Check sheet for the modelled part. Datum: model origin and axes. Units: mm. A direction names the side the tool comes from. Round coordinates to 2 decimals unless told otherwise and drop trailing zeros. Write each loop counter-clockwise with the first axis right and the second up, starting at its lowest first coordinate (ties: lowest second). Pieces come first, ordered by that corner, then holes. Notation, with made-up numbers: M 21.5,89 L 33.5,89 A15 ccw 33.5,108 Z; hole C 39,69.5 d3. An arc over 180 degrees is marked long. Answer in a Markdown table with one row per item.
```python
from build123d import *

# Parameters (mm, degrees)
SKETCH1_R      = 1.75
EXTRUDE1_DEPTH = 3


with BuildPart() as part:
    # Sketch1 → Extrude1 (new body)
    with BuildSketch(Plane.XY):
        with BuildLine():
            Line((-4, -50.76970061), (-4, -54.401493546))
            ThreePointArc((-4, -54.401493546), (-5.018660435, -56.654112805), (-7.382862352, -57.376962655))
            ThreePointArc((-7.382862352, -57.376962655), (-8.491134253, -57.223449207), (-9.596229972, -57.048530834))
            ThreePointArc((-9.596229972, -57.048530834), (-12.103146033, -55.797735176), (-13.484767706, -53.360474528))
            ThreePointArc((-13.484767706, -53.360474528), (-14.450357204, -51.517657712), (-16.210841333, -50.409040319))
            ThreePointArc((-16.210841333, -50.409040319), (0, 57.25), (16.210841333, -50.409040319))
            ThreePointArc((16.210841333, -50.409040319), (14.450357204, -51.517657712), (13.484767706, -53.360474528))
            ThreePointArc((13.484767706, -53.360474528), (12.103146033, -55.797735176), (9.596229972, -57.048530834))
            ThreePointArc((9.596229972, -57.048530834), (8.491134253, -57.223449207), (7.382862352, -57.376962655))
            ThreePointArc((7.382862352, -57.376962655), (5.018660435, -56.654112805), (4, -54.401493546))
            Line((4, -54.401493546), (4, -50.76970061))
            ThreePointArc((4, -50.76970061), (4.738444308, -48.79856747), (6.590243902, -47.797815696))
            ThreePointArc((6.590243902, -47.797815696), (0, 48.25), (-6.590243902, -47.797815696))
            ThreePointArc((-6.590243902, -47.797815696), (-4.738444308, -48.79856747), (-4, -50.76970061))
        make_face()
        with Locations((-8.8, -52.315031301)):
            Circle(SKETCH1_R, mode=Mode.SUBTRACT)
        with Locations((8.8, -52.315031301)):
            Circle(SKETCH1_R, mode=Mode.SUBTRACT)
    extrude(amount=EXTRUDE1_DEPTH)


solid = part.part
```
1. Draft check along X on faces 1 (the face through (-14.43, -51.54, 1.48)), 2 (the face through (14.47, -51.496, 1.479)), 3 (the face through (-4.758, -48.776, 1.479)). Enter one of: +X half, -X half, draft (parallel to the pull), parting line (faces both ways), or undercut.
Found:
| item | result |
|---|---|
| face 1 | -X half |
| face 2 | +X half |
| face 3 | undercut |
2. Section check D-D, the plane x = 0. Record the cut outline in (y, z), and give its area (3 significant figures).
Found:
| item | result |
|---|---|
| outline | M 48.25,0 L 57.25,0 L 57.25,3 L 48.25,3 Z |
| area | 27.0 mm2 |
3. Section check A-A, the plane x = 29. Record the cut outline in (y, z), and give its area (3 significant figures).
Found:
| item | result |
|---|---|
| outline | M -44.59,0 L -38.56,0 L -38.56,3 L -44.59,3 Z; M 38.56,0 L 48.99,0 L 48.99,3 L 38.56,3 Z |
| area | 49.4 mm2 |
4. Access from +Z, -Z, +X, -X, +Y, -Y to the whole of each face (thin tool, end or side, straight path). Record for faces 4 (the face through (-4, -53, 1)), 5 (the face through (12, 47, 3)), 6 (the face through (4.72, -48.82, 1.48)).
Found:
| item | result |
|---|---|
| face 4 | +Z, -Z, -Y |
| face 5 | +Z, +X, -X, +Y, -Y |
| face 6 | +Z, -Z |
5. Section check C-C, the plane z = 1.2. Record the cut outline in (x, y).
Found:
| item | result |
|---|---|
| outline | M -16.21,-50.41 A4 cw -13.48,-53.36 A4.8 ccw -9.6,-57.05 A57.85 ccw -7.38,-57.38 A3 ccw -4,-54.4 L -4,-50.77 A3 ccw -6.59,-47.8 A48.25 cw long 6.59,-47.8 A3 ccw 4,-50.77 L 4,-54.4 A3 ccw 7.38,-57.38 A57.85 ccw 9.6,-57.05 A4.8 ccw 13.48,-53.36 A4 cw 16.21,-50.41 A55.05 ccw long Z; hole C -8.8,-52.32 d3.5; hole C 8.8,-52.32 d3.5 |
6. Scan lines: L1, parallel to Y at x = -8.8, z = 2.2; L2, parallel to Y at x = -9, z = 0.45; L3, parallel to Y at x = 21.5, z = 2.35. Record each from-to range of solid material in increasing order.
Found:
| item | result |
|---|---|
| L1 | y = -57.18 to -54.07, -50.57 to -47.44, 47.44 to 56.54 |
| L2 | y = -57.15 to -54.05, -50.58 to -47.4, 47.4 to 56.51 |
| L3 | y = -48.48 to -43.2, 43.2 to 52.88 |
7. Section check B-B, the plane y = 21. Record the cut outline in (x, z).
Found:
| item | result |
|---|---|
| outline | M -51.74,0 L -43.44,0 L -43.44,3 L -51.74,3 Z; M 43.44,0 L 51.74,0 L 51.74,3 L 43.44,3 Z |
